CAD build for the part. Positions are in the model's coordinates, mm. Give positions to 0.01 mm unless a question says otherwise; leave off trailing zeros. Loops run counter-clockwise (first coordinate to the right, second up) from the corner with the lowest first, then second, coordinate; pieces in that order, holes last.
Autodesk Inventor part; units mm, degrees
ref_plane "YZ Plane" through (0, 0, 0) normal (1, 0, 0) x (0, 1, 0)
ref_plane "XZ Plane" through (0, 0, 0) normal (0, 1, 0) x (-1, 0, 0)
ref_plane "XY Plane" through (0, 0, 0) normal (0, 0, 1) x (1, 0, 0)
sketch "Sketch1" plane through (0, 0, 0) normal (0, 1, 0) x (-1, 0, 0)
  line L0 (0, -7.3323) -> (-6.35, -3.6662)
  line L1 (-6.35, -3.6662) -> (-6.35, 3.6662)
  line L2 (-6.35, 3.6662) -> (0, 7.3323)
  line L3 (0, 7.3323) -> (6.35, 3.6662)
  line L4 (6.35, 3.6662) -> (6.35, -3.6662)
  line L5 (6.35, -3.6662) -> (0, -7.3323)
  circle A0 centre (0, 0) radius 2.0193
  point P0 (-3.175, 5.4993)
  point P1 (6.35, 0)
  dimension "d0" = 12.7
  dimension "d1" = 4.0386
extrude "Extrusion1" add sketch "Sketch1" along normal blind 39.878
thread "Thread1"
properties part number "Gearbox4_003_Hexshaft"
1. Saw through at B-B, the plane z = 0. List the corners of the cut face in (x, y).
Responses:
outline: (-6.35, 0) - (-2.02, 0) - (-2.02, 39.88) - (-6.35, 39.88) - close; (2.02, 0) - (6.35, 0) - (6.35, 39.88) - (2.02, 39.88) - close
2. Saw through at D-D, the plane x = 4. List the corners of the cut face in (y, z).
Responses:
outline: (0, -5.02) - (39.88, -5.02) - (39.88, 5.02) - (0, 5.02) - close
3. Probe line 1 along Z through (x, y) = (-1, 20); line 2 along Z through (x, y) = (0, 21); line 3 along Z through (x, y) = (4, 37.5). List the from-to ranges inside material, lowest first.
Responses:
line 1: z = -6.75 to -1.75, 1.75 to 6.75
line 2: z = -7.33 to -2.02, 2.02 to 7.33
line 3: z = -5.02 to 5.02
4. Drop flat-ended pins along their axis: pin 1 (1 mm diameter, centred on x = -1.5, y = 6, fed in from -Z); pin 2 (1 mm diameter, centred on x = 4.5, y = 6, fed in from -Z); pin 3 (3 mm diameter, centred on y = 11.5, z = 5.5, fed in from -X). Give the stop position or say it passes through.
Responses:
pin 1: stops at z = -6.75
pin 2: stops at z = -5.02
pin 3: stops at x = -5.77
5. Saw through at A-A, the plane y = 14.5. List the corners of the cut face in (x, z).
Responses:
outline: (-6.35, -3.67) - (0, -7.33) - (6.35, -3.67) - (6.35, 3.67) - (0, 7.33) - (-6.35, 3.67) - close; hole circle Ø4.04 at (0, 0)
6. Saw through at C-C, the plane x = 1.25. List the corners of the cut face in (y, z), and give its area (3 significant figures).
Responses:
outline: (0, -6.61) - (39.88, -6.61) - (39.88, -1.59) - (0, -1.59) - close; (0, 1.59) - (39.88, 1.59) - (39.88, 6.61) - (0, 6.61) - close
area: 401 mm2
